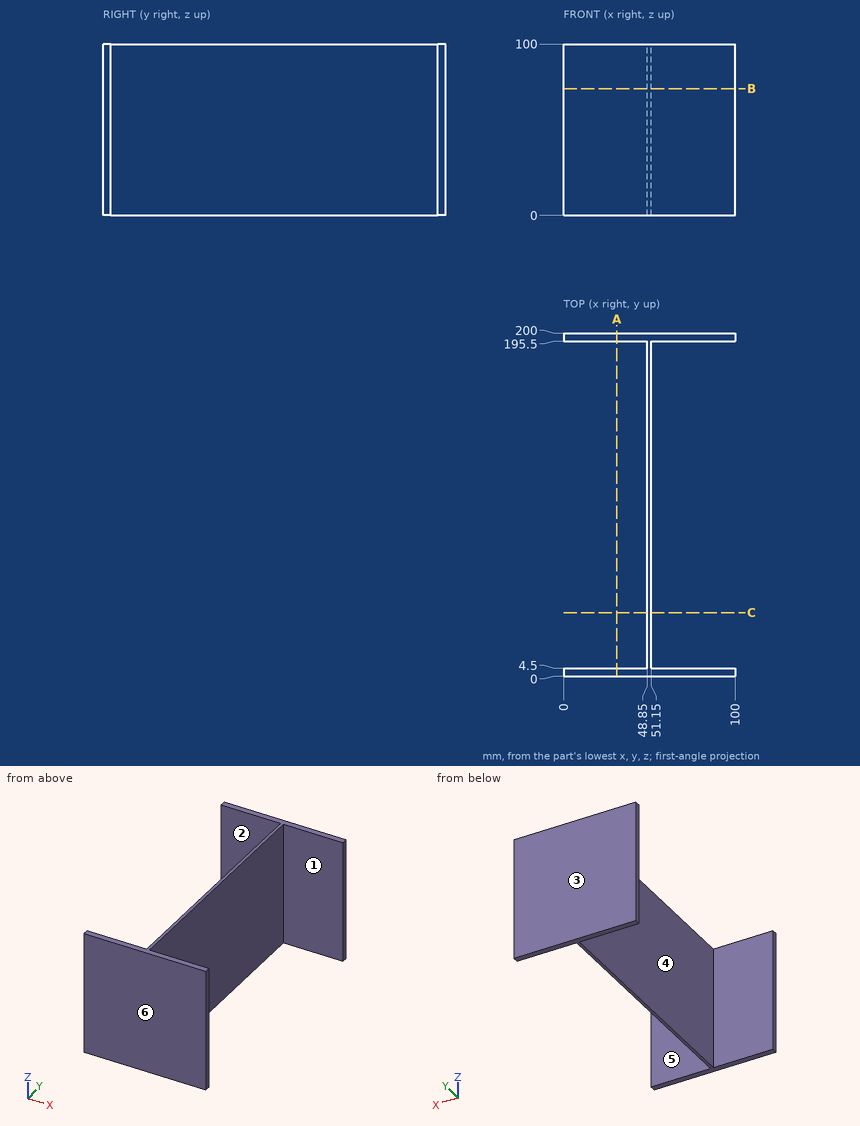
Study the drawing (mm; zero at the part's minimum x, y, z) and answer. A direction names the side the tool comes from. Round coordinates to 2 decimals unless told otherwise and drop trailing zeros. Write each loop counter-clockwise with the first axis right and the second up, starting at its lowest first coordinate (ties: lowest second). Pieces come first, ordered by that corner, then holes. Notation, with made-up numbers: (-33, -13) - (20, -13) arc R38 ccw to (20, 25) - close; hole circle Ø4 at (-25, 73). An arc over 180 degrees is marked (long way). Return JSON: item names as keys, results as strings. Group by question number.
Q1. For the marked faces 1 and 2, determine the directions among +Z, -Z, +X, -X, +Y, -Y from which every point of the face is accessible in a straight line to the end or side of a thin tool.
Q2. The mould has two halves that part along Y. Classify the marked faces 3, 4, 5 and 6: released by +Y, released by -Y, zero draft, split by the parting line, or undercut.
Q3. The part is cut by section B-B on z = 74. Write down the section's boundary in (x, y).
Q4. The part is cut by section A-A on x = 31. Write down the section's boundary in (y, z).
Q5. Each of these flat-tipped pins is pushed along its axis until it touches: pin 1 Ø8 at (y, z) = (95, 77.5) entering from +X; pin 2 Ø12 at (x, y) = (62, 61) entering from -Z. Where does it stop, or does it pass through?
Q6. The part is cut by section C-C on y = 37. Write down the section's boundary in (x, z).
Q7. Find the intervals of material crossed by L1, parallel to Y at x = 59.5, z = 49; L2, parallel to X at y = 84.5, z = 83, in increasing order.
Solved:
{
 "1": {"face 1": "+Z, -Z, +X", "face 2": "+Z, -Z, -X"},
 "2": {"face 3": "released by +Y", "face 4": "undercut", "face 5": "undercut", "face 6": "released by -Y"},
 "3": {"outline": "(0, 0) - (100, 0) - (100, 4.5) - (51.15, 4.5) - (51.15, 195.5) - (100, 195.5) - (100, 200) - (0, 200) - (0, 195.5) - (48.85, 195.5) - (48.85, 4.5) - (0, 4.5) - close"},
 "4": {"outline": "(0, 0) - (4.5, 0) - (4.5, 100) - (0, 100) - close; (195.5, 0) - (200, 0) - (200, 100) - (195.5, 100) - close"},
 "5": {"pin 1": "x = 51.15", "pin 2": "through"},
 "6": {"outline": "(48.85, 0) - (51.15, 0) - (51.15, 100) - (48.85, 100) - close"},
 "7": {"L1": "0 to 4.5, 195.5 to 200", "L2": "48.85 to 51.15"}
}
